Read the model definition and answer for the solid it produces. Units are mm, in the model's axes. Face numbers are marked on the shaded views. A direction names the side the tool comes from. Give positions to 0.01 mm unless a question says otherwise; leave off trailing zeros. Order: outer loops, then holes, each group sorted by start corner. A loop starts at its lowest first (then second) coordinate and runs counter-clockwise, first axis right, second up. Notation, with made-up numbers: M -0.75,-23.75 L 23.25,-23.75 A12 ccw 23.25,-0.75 Z; hole C -16.5,12 d2. An arc over 180 degrees is marked long. One line per item, written item: value.
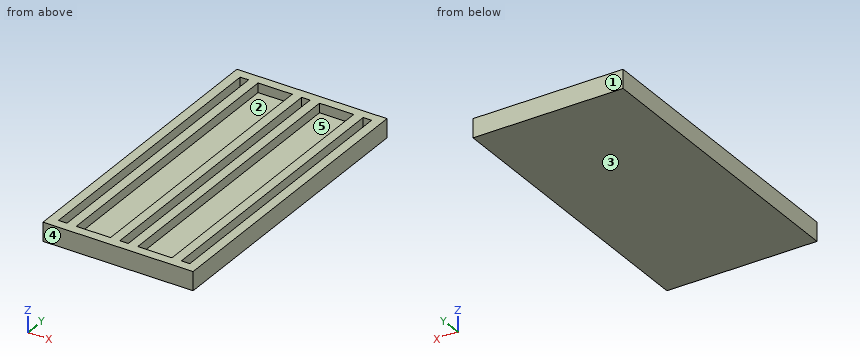
from build123d import *

# Parameters (mm, degrees)
F1_DEPTH      = 30
F1_DEPTH_BACK = 30
F2_W          = 32
F2_H          = 4
F3_DEPTH      = 2
F4_W          = 32
F4_H          = 4
F5_DEPTH      = 2


with BuildPart() as f1:
    # F0 (on Front) → F1 (new body, two sides)
    with BuildSketch(Plane.XZ) as f1_sk:
        Polygon((-16, 4), (-16, 0), (16, 0), (16, 4), (14, 4), (14, 2), (12.2, 2), (12.2, 4), (10.2, 4), (10.2, 2), (2.9, 2), (2.9, 4), (0.9, 4), (0.9, 2), (-0.9, 2), (-0.9, 4), (-2.9, 4), (-2.9, 2), (-10.2, 2), (-10.2, 4), (-12.2, 4), (-12.2, 2), (-14, 2), (-14, 4), align=None)
    extrude(amount=F1_DEPTH)
    extrude(f1_sk.sketch, amount=-F1_DEPTH_BACK)

    # F2 (on face) → F3 (join)
    with BuildSketch(Plane.XZ.offset(30)):
        with Locations((0, 2)):
            Rectangle(F2_W, F2_H)
    extrude(amount=F3_DEPTH)

    # F4 (on face) → F5 (join)
    with BuildSketch(Plane(origin=(0, 30, 0), x_dir=(-1, 0, 0), z_dir=(0, 1, 0))):
        with Locations((0, 2)):
            Rectangle(F4_W, F4_H)
    extrude(amount=F5_DEPTH)


solid = f1.part
1) This flat-tipped pin is pushed along its axis until it touches: pin 1 Ø0.5 at (x, y) = (0.5, 9) entering from +Z. Where does it stop, or does it pass through?
Reported:
pin 1: stops at z = 2
2) Determine the mould class of the marked faces 1, 2 and 3 for opening direction Y: +Y half, -Y half, draft (parallel to the pull), parting line (faces both ways), or undercut.
Reported:
face 1: +Y half
face 2: undercut
face 3: draft
3) Consider probe 1 along X at (y, z) = (24, 3.35); probe 2 along Y at (x, z) = (-9, 3.2); probe 3 along Z at (x, y) = (-7, 8.5). Determine where each line is inside the solid, lowest interval first.
Reported:
probe 1: x = -16 to -14, -12.2 to -10.2, -2.9 to -0.9, 0.9 to 2.9, 10.2 to 12.2, 14 to 16
probe 2: y = -32 to -30, 30 to 32
probe 3: z = 0 to 2
4) Find section C-C, the plane y = -8. Write down the section's boundary in (x, z), plus the area to 3 significant figures.
Reported:
outline: M -16,0 L 16,0 L 16,4 L 14,4 L 14,2 L 12.2,2 L 12.2,4 L 10.2,4 L 10.2,2 L 2.9,2 L 2.9,4 L 0.9,4 L 0.9,2 L -0.9,2 L -0.9,4 L -2.9,4 L -2.9,2 L -10.2,2 L -10.2,4 L -12.2,4 L -12.2,2 L -14,2 L -14,4 L -16,4 Z
area: 88.0 mm^2
5) Find section A-A, the plane z = 3.1. Write down the section's boundary in (x, y).
Reported:
outline: M -16,-32 L 16,-32 L 16,32 L -16,32 Z; hole M -14,-30 L -12.2,-30 L -12.2,30 L -14,30 Z; hole M -10.2,-30 L -2.9,-30 L -2.9,30 L -10.2,30 Z; hole M -0.9,-30 L 0.9,-30 L 0.9,30 L -0.9,30 Z; hole M 2.9,-30 L 10.2,-30 L 10.2,30 L 2.9,30 Z; hole M 12.2,-30 L 14,-30 L 14,30 L 12.2,30 Z
6) Which of the six approach directions +Z, -Z, +X, -X, +Y, -Y give full straight-line access (tool end or side, diameter ignored) to the marked faces 4 and 5?
Reported:
face 4: +Z, -Z, +X, -X, -Y
face 5: +Z
7) Find section B-B, the plane x = -9. Write down the section's boundary in (y, z).
Reported:
outline: M -32,0 L 32,0 L 32,4 L 30,4 L 30,2 L -30,2 L -30,4 L -32,4 Z
